The listing builds one solid part. Answer for the finished solid, in the listing's coordinates (mm). Face numbers are marked on the shaded views. A direction names the side the tool comes from. Give positions to 0.01 mm unless a question says otherwise; leave off trailing zeros. Order: outer loops, then holes, each group sorted by start corner. A loop starts at its lowest first (then second) coordinate and runs counter-clockwise, first axis right, second up. Notation, with made-up numbers: (35, 2.5) - (91, 2.5) arc R33 ccw to (91, 40.5) - close; hole circle Ø7 at (49.25, 16). An arc over 180 degrees is marked (long way). Answer as a JSON object with one key per item and string values. Group by question number.
Q1. For the marked faces 4, 5 and 6, determine the directions among +Z, -Z, +X, -X, +Y, -Y from which every point of the face is accessible in a straight line to the end or side of a thin tool.
Q2. A cutting plane is placed at A-A, the plane y = -2.75. Count the separate pieces of the cut face and the enclosed holes in it, and give its area (3 significant figures).
Q3. Consider line 1 (Y direction, x = -4, z = -9); line 2 (X direction, y = -4.5, z = -9.5); line 3 (X direction, y = -4.75, z = 11). Determine where each line is inside the solid, lowest interval first.
Q4. A cutting plane is placed at B-B, the plane z = -12. Give the vertices of the cut face in (x, y), and give its area (3 significant figures).
Q5. Given pin 1 (3 mm diameter, centred on x = -7, y = -6.5, fed in from +Z); pin 2 (2 mm diameter, centred on x = 1, y = -5.5, fed in from +Z); pin 3 (1.5 mm diameter, centred on y = -3.5, z = -13, fed in from -X), each flat-ended and moving along its own axis, determine where each tip first touches the part or whether it passes through.
Q6. A cutting plane is placed at C-C, the plane y = -6. Give the vertices of the cut face in (x, z).
Q7. The mould has two halves that part along X. Classify the marked faces 1, 2 and 3: released by +X, released by -X, zero draft, split by the parting line, or undercut.
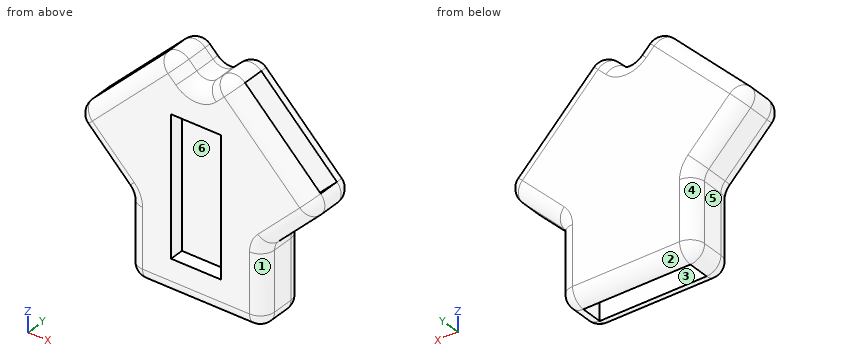
from build123d import *

# Parameters (mm, degrees)
F1_DEPTH  = 7
F2_W      = 15
F2_H      = 3
F3_DEPTH  = 25
F4_W      = 15
F4_H      = 3
F5_DEPTH  = 19.6
F6_W      = 3
F6_H      = 15
F7_DEPTH  = 21.3
F8_R      = 1.99999
F9_W      = 7
F9_H      = 19.3284271247
F10_DEPTH = 2


# Not quite as in the source:
# - a fillet or chamfer is up to 0.001 mm smaller than in the source, because OpenCascade refuses the exact size


with BuildPart() as f1:
    # F0 (on Front) → F1 (new body)
    with BuildSketch(Plane.XZ):
        Polygon((0, 9.5), (-9.5, 0), (9.5, 0), align=None)
        Polygon((9.5, 0), (-9.5, 0), (-9.5, -7.8700576851), (-9.5, -19), (9.5, -19), (9.5, -7.8700576851), align=None)
        Polygon((-9.5, -7.8700576851), (-9.5, 0), (0, 9.5), (-3.9350288425, 13.4350288425), (-17.3700576851, 0), align=None)
        Polygon((0, 9.5), (9.5, 0), (9.5, -7.8700576851), (17.3700576851, 0), (3.9350288425, 13.4350288425), align=None)
    extrude(amount=F1_DEPTH)

    # F2 (on face) → F3 (cut)
    with BuildSketch(Plane(origin=(0, 0, -19), x_dir=(1, 0, 0), z_dir=(0, 0, -1))):
        with Locations((0, 3.5)):
            Rectangle(F2_W, F2_H)
    extrude(amount=-F3_DEPTH, mode=Mode.SUBTRACT)

    # F4 (on face) → F5 (cut)
    with BuildSketch(Plane(origin=(8.6850288425, 0, 8.6850288425), x_dir=(0.7071067812, 0, -0.7071067812), z_dir=(0.7071067812, 0, 0.7071067812))):
        with Locations((2.7824855787, -3.5)):
            Rectangle(F4_W, F4_H)
    extrude(amount=-F5_DEPTH, mode=Mode.SUBTRACT)

    # F6 (on face) → F7 (cut)
    with BuildSketch(Plane(origin=(-8.6850288425, 0, 8.6850288425), x_dir=(0, -1, 0), z_dir=(-0.7071067812, 0, 0.7071067812))):
        with Locations((3.5, -2.7824855787)):
            Rectangle(F6_W, F6_H)
    extrude(amount=-F7_DEPTH, mode=Mode.SUBTRACT)

    # F8 (radius 2 in the source; OpenCascade refuses exactly that, so slightly less here)
    f8_edges = [f1.edges().sort_by_distance(p)[0] for p in [
        (-9.5, -7, -13.435029),
        (-13.435029, -7, -3.935029),
        (-13.435029, 0, -3.935029),
        (-9.5, 0, -13.435029),
        (0, -7, -19),
        (0, 0, -19),
        (-9.5, -3.5, -19),
        (9.5, -3.5, -19),
        (9.5, -7, -13.435029),
        (9.5, 0, -13.435029),
        (13.435029, 0, -3.935029),
        (13.435029, -7, -3.935029),
        (17.370058, -3.5, 0),
        (10.652543, -7, 6.717514),
        (3.935029, -3.5, 13.435029),
        (10.652543, 0, 6.717514),
        (1.967514, 0, 11.467514),
        (-1.967514, 0, 11.467514),
        (-1.967514, -7, 11.467514),
        (1.967514, -7, 11.467514),
        (-10.652543, -7, 6.717514),
        (-3.935029, -3.5, 13.435029),
        (-10.652543, 0, 6.717514),
        (-17.370058, -3.5, 0),
        (0, -3.5, 9.5),
        (-9.5, -3.5, -7.870058),
        (9.5, -3.5, -7.870058),
    ]]
    fillet(f8_edges, radius=F8_R)

    # F9 (on face) → F10 (cut)
    with BuildSketch(Plane.XZ.offset(7)):
        with Locations((0, -4.3357864376)):
            Rectangle(F9_W, F9_H)
    extrude(amount=-F10_DEPTH, mode=Mode.SUBTRACT)


solid = f1.part
Reply:
{
 "1": {"face 4": "-Z, -X, +Y", "face 5": "-Z, -X, +Y, -Y", "face 6": "none"},
 "2": {"separate pieces": "3", "enclosed holes": "0", "area": "114 mm^2"},
 "3": {"line 1": "y = -7 to -5, -2 to 0", "line 2": "x = -9.5 to -7.5, 7.5 to 9.5", "line 3": "x = -4.33 to -1.5, 1.5 to 4.33"},
 "4": {"outline": "(-9.5, -5) arc R2 ccw to (-7.5, -7) - (-3.5, -7) - (-3.5, -5) - (-7.5, -5) - (-7.5, -2) - (7.5, -2) - (7.5, -5) - (3.5, -5) - (3.5, -7) - (7.5, -7) arc R2 ccw to (9.5, -5) - (9.5, -2) arc R2 ccw to (7.5, 0) - (-7.5, 0) arc R2 ccw to (-9.5, -2) - close", "area": "70.6 mm^2"},
 "5": {"pin 1": "stops at z = 11.46", "pin 2": "stops at z = 11.45", "pin 3": "stops at x = -9.5"},
 "6": {"outline": "(-15.77, -1.22) - (-9.9, -7.09) arc R2.27 cw to (-9.23, -8.7) - (-9.23, -17) arc R1.73 ccw to (-7.5, -18.73) - (7.5, -18.73) arc R1.73 ccw to (9.23, -17) - (9.23, -8.7) arc R2.27 cw to (9.9, -7.09) - (15.77, -1.22) arc R1.73 ccw to (15.77, 1.22) - (5.16, 11.83) arc R1.73 ccw to (2.71, 11.83) - (1.6, 10.72) arc R2.27 cw to (-1.6, 10.72) - (-2.71, 11.83) arc R1.73 ccw to (-5.16, 11.83) - (-15.77, 1.22) arc R1.73 ccw to start; hole (-3.5, -14) - (3.5, -14) - (3.5, 5.33) - (-3.5, 5.33) - close"},
 "7": {"face 1": "released by +X", "face 2": "zero draft", "face 3": "undercut"}
}
